from build123d import *

# Parameters (mm, degrees)
SKETCH1_W           = 80
SKETCH1_H           = 40
BOSS_EXTRUDE1_DEPTH = 15
FILLET2_R           = 1
SKETCH2_W           = 6.044627726
SKETCH2_H           = 2.581559758
BOSS_EXTRUDE2_DEPTH = 1
SKETCH3_R           = 1.362138451
CUT_EXTRUDE1_DEPTH  = 1
SKETCH4_R           = 1.077712871
CUT_EXTRUDE2_DEPTH  = 1
SKETCH5_W           = 2.171547326
SKETCH5_H           = 5.220065687
CUT_EXTRUDE3_DEPTH  = 2
SKETCH6_W           = 2.380349953
SKETCH6_H           = 7.349852488
CUT_EXTRUDE4_DEPTH  = 3
FILLET3_R           = 1
SKETCH7_R           = 0.422381203
BOSS_EXTRUDE3_DEPTH = 0.6


with BuildPart() as part:
    # Sketch1 → Boss-Extrude1 (new body)
    with BuildSketch(Plane.XY):
        with Locations((30.786516854, -9.438202247)):
            Rectangle(SKETCH1_W, SKETCH1_H)
    extrude(amount=BOSS_EXTRUDE1_DEPTH)

    # Fillet2
    fillet2_edges = [part.edges().sort_by_distance(p)[0] for p in [
        (70.786516854, -9.438202247, 15),
        (30.786516854, 10.561797753, 15),
        (-9.213483146, -9.438202247, 15),
        (30.786516854, 10.561797753, 0),
        (70.786516854, -9.438202247, 0),
        (30.786516854, -29.438202247, 0),
        (-9.213483146, -9.438202247, 0),
        (-9.213483146, 10.561797753, 7.5),
        (70.786516854, 10.561797753, 7.5),
        (70.786516854, -29.438202247, 7.5),
        (-9.213483146, -29.438202247, 7.5),
        (30.786516854, -29.438202247, 15),
    ]]
    fillet(fillet2_edges, radius=FILLET2_R)

    # Sketch2 → Boss-Extrude2 (add)
    with BuildSketch(Plane(origin=(0, 10.561797753, 0), x_dir=(1, 0, 0), z_dir=(0, 1, 0))):
        with Locations((5.789462611, -7.027763459)):
            Rectangle(SKETCH2_W, SKETCH2_H)
    extrude(amount=BOSS_EXTRUDE2_DEPTH)

    # Sketch3 → Cut-Extrude1 (cut)
    with BuildSketch(Plane.XY.offset(15)):
        with Locations((-1.514462559, -18.319968197)):
            Circle(SKETCH3_R)
        with Locations((-1.514462559, -13.319968197)):
            Circle(SKETCH3_R)
        with Locations((-1.514462559, -8.319968197)):
            Circle(SKETCH3_R)
        with Locations((-1.514462559, -3.319968197)):
            Circle(SKETCH3_R)
    extrude(amount=-CUT_EXTRUDE1_DEPTH, mode=Mode.SUBTRACT)

    # Sketch4 → Cut-Extrude2 (cut)
    with BuildSketch(Plane.ZY.offset(9.213483146)):
        with Locations((6.831831592, 4.174602759)):
            Circle(SKETCH4_R)
    extrude(amount=-CUT_EXTRUDE2_DEPTH, mode=Mode.SUBTRACT)

    # Sketch5 → Cut-Extrude3 (cut)
    with BuildSketch(Plane(origin=(70.786516854, 0, 0), x_dir=(0, 0, -1), z_dir=(1, 0, 0))):
        with Locations((-3.591405193, 3.151469884)):
            Rectangle(SKETCH5_W, SKETCH5_H)
        with Locations((-11.091405193, 3.151469884)):
            Rectangle(SKETCH5_W, SKETCH5_H)
    extrude(amount=-CUT_EXTRUDE3_DEPTH, mode=Mode.SUBTRACT)

    # Sketch6 → Cut-Extrude4 (cut)
    with BuildSketch(Plane(origin=(70.786516854, 0, 0), x_dir=(0, 0, -1), z_dir=(1, 0, 0))):
        with Locations((-7.896724993, -20.380586234)):
            Rectangle(SKETCH6_W, SKETCH6_H)
    extrude(amount=-CUT_EXTRUDE4_DEPTH, mode=Mode.SUBTRACT)

    # Fillet3
    fillet3_edges = [part.edges().sort_by_distance(p)[0] for p in [
        (67.786516854, -20.380586234, 9.086899969),
        (69.286516854, -24.055512478, 9.086899969),
        (67.786516854, -16.70565999, 7.896724992),
        (69.286516854, -16.70565999, 9.086899969),
        (67.786516854, -20.380586234, 6.706550016),
        (69.286516854, -16.70565999, 6.706550016),
        (67.786516854, -24.055512478, 7.896724992),
        (69.286516854, -24.055512478, 6.706550016),
        (70.786516854, -20.380586234, 9.086899969),
        (70.786516854, -24.055512478, 7.896724992),
        (70.786516854, -20.380586234, 6.706550016),
        (70.786516854, -16.70565999, 7.896724992),
    ]]
    fillet(fillet3_edges, radius=FILLET3_R)

    # Sketch7 → Boss-Extrude3 (add)
    with BuildSketch(Plane.XY.offset(15)):
        with Locations((63.276390883, -22.727509248)):
            Circle(SKETCH7_R)
        with Locations((64.276390883, -22.727509248)):
            Circle(SKETCH7_R)
        with Locations((65.276390883, -22.727509248)):
            Circle(SKETCH7_R)
        with Locations((66.276390883, -22.727509248)):
            Circle(SKETCH7_R)
        with Locations((67.276390883, -22.727509248)):
            Circle(SKETCH7_R)
        with Locations((64.276390883, -21.727509248)):
            Circle(SKETCH7_R)
        with Locations((65.276390883, -21.727509248)):
            Circle(SKETCH7_R)
        with Locations((66.276390883, -21.727509248)):
            Circle(SKETCH7_R)
        with Locations((67.276390883, -21.727509248)):
            Circle(SKETCH7_R)
        with Locations((64.276390883, -20.727509248)):
            Circle(SKETCH7_R)
        with Locations((65.276390883, -20.727509248)):
            Circle(SKETCH7_R)
        with Locations((66.276390883, -20.727509248)):
            Circle(SKETCH7_R)
        with Locations((67.276390883, -20.727509248)):
            Circle(SKETCH7_R)
        with Locations((64.276390883, -19.727509248)):
            Circle(SKETCH7_R)
        with Locations((65.276390883, -19.727509248)):
            Circle(SKETCH7_R)
        with Locations((66.276390883, -19.727509248)):
            Circle(SKETCH7_R)
        with Locations((67.276390883, -19.727509248)):
            Circle(SKETCH7_R)
        with Locations((64.276390883, -18.727509248)):
            Circle(SKETCH7_R)
        with Locations((65.276390883, -18.727509248)):
            Circle(SKETCH7_R)
        with Locations((66.276390883, -18.727509248)):
            Circle(SKETCH7_R)
        with Locations((67.276390883, -18.727509248)):
            Circle(SKETCH7_R)
        with Locations((64.276390883, -17.727509248)):
            Circle(SKETCH7_R)
        with Locations((65.276390883, -17.727509248)):
            Circle(SKETCH7_R)
        with Locations((66.276390883, -17.727509248)):
            Circle(SKETCH7_R)
        with Locations((67.276390883, -17.727509248)):
            Circle(SKETCH7_R)
        with Locations((64.276390883, -16.727509248)):
            Circle(SKETCH7_R)
        with Locations((65.276390883, -16.727509248)):
            Circle(SKETCH7_R)
        with Locations((66.276390883, -16.727509248)):
            Circle(SKETCH7_R)
        with Locations((67.276390883, -16.727509248)):
            Circle(SKETCH7_R)
        with Locations((63.276390883, -21.727509248)):
            Circle(SKETCH7_R)
        with Locations((63.276390883, -20.727509248)):
            Circle(SKETCH7_R)
        with Locations((63.276390883, -19.727509248)):
            Circle(SKETCH7_R)
        with Locations((63.276390883, -18.727509248)):
            Circle(SKETCH7_R)
        with Locations((63.276390883, -17.727509248)):
            Circle(SKETCH7_R)
        with Locations((63.276390883, -16.727509248)):
            Circle(SKETCH7_R)
    extrude(amount=BOSS_EXTRUDE3_DEPTH)


solid = part.part
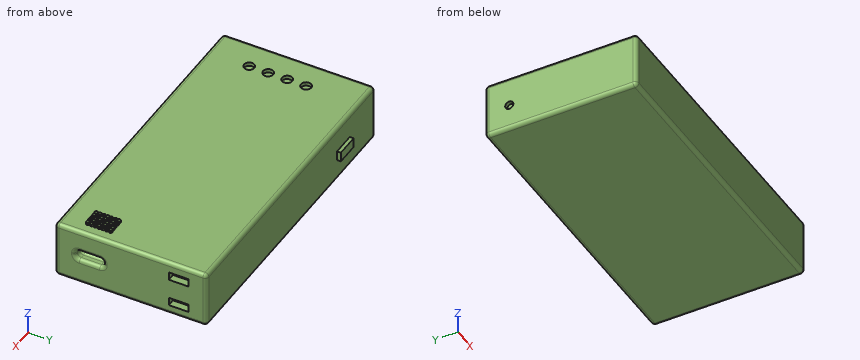
The model under review builds one solid part; all positions refer to its coordinate system, in mm. Round coordinates to 2 decimals unless told otherwise and drop trailing zeros. Loops run counter-clockwise (first coordinate to the right, second up) from the corner with the lowest first, then second, coordinate; pieces in that order, holes last. Notation, with made-up numbers: (27.25, -8.5) -> (50.25, -8.5) arc R22 cw to (50.25, 2.5) -> close; hole circle Ø10 at (-34.5, -0.75). An arc over 180 degrees is marked (long way). One line per question, with ' | ' between items. Start each with the question number.
Item 1: Add section B-B, the plane y = 7.5. Write out the cut boundary in (x, z), then the cut area to 3 significant figures.
Item 2: For pin 1 (0.8 mm diameter, centred on y = 11, z = 7, fed in from +X); pin 2 (0.8 mm diameter, centred on x = 5, y = 11, fed in from -Z); pin 3 (3 mm diameter, centred on x = -1.5, y = -3, fed in from +Z), all flat-tipped, find the tip position at first contact; note any pin that passes through.
Item 3: Add section A-A, the plane x = 58. Write out the cut boundary in (y, z), then the cut area to 3 significant figures.
Item 4: Wall thickness on line 1 along X through (y, z) = (-21, 15.25); line 2 along Z through (x, y) = (35, 0); line 3 along Y through (x, z) = (16, 3.5): over which ranges is each line inside the solid? List them lowest first. Write a range as [from, to].
Return value:
1) outline: (-9.21, 1) arc R1 ccw to (-8.21, 0) -> (69.79, 0) arc R1 ccw to (70.79, 1) -> (70.79, 14) arc R1 ccw to (69.79, 15) -> (-8.21, 15) arc R1 ccw to (-9.21, 14) -> close | area: 1,200 mm2
2) pin 1: stops at x = 8.81 | pin 2: stops at z = 5.74 | pin 3: stops at z = 15
3) outline: (-29.44, 1) arc R1 ccw to (-28.44, 0) -> (9.56, 0) arc R1 ccw to (10.56, 1) -> (10.56, 14) arc R1 ccw to (9.56, 15) -> (-28.44, 15) arc R1 ccw to (-29.44, 14) -> close | area: 599 mm2
4) line 1: x = [62.95, 63.6], [63.95, 64.6], [64.95, 65.6], [65.95, 66.6], [66.95, 67.6] | line 2: z = [0, 15] | line 3: y = [-29.44, 10.56]
